from build123d import *

# Parameters (mm, degrees)
BOSS_EXTRUDE1_DEPTH = 10
CHAMFER1_SIZE       = 7.802060087
CHAMFER1_SIZE_2     = 10
BOSS_EXTRUDE2_DEPTH = 20
SKETCH7_R           = 1.5
CUT_EXTRUDE1_DEPTH  = 20
CUT_EXTRUDE3_DEPTH  = 20
FILLET5_R           = 20
FILLET6_R           = 10
SKETCH10_W          = 5.3
SKETCH10_H          = 4.24
CUT_EXTRUDE4_DEPTH  = 273.805653344
SKETCH11_W          = 3.75
SKETCH11_H          = 144.691495626
CUT_EXTRUDE5_DEPTH  = 370.011076387
BOSS_EXTRUDE4_DEPTH = 12.5
SKETCH12_W          = 2
SKETCH12_H          = 1.5
CUT_EXTRUDE6_DEPTH  = 144.691496
CUT_EXTRUDE7_DEPTH  = 273.805653344
SKETCH15_W          = 8
SKETCH15_H          = 10
CUT_EXTRUDE8_DEPTH  = 234.574560204
SKETCH16_R          = 1.45
CUT_EXTRUDE9_DEPTH  = 230.270963046


with BuildPart() as part:
    # Sketch2 → Boss-Extrude1 (new, symmetric)
    with BuildSketch(Plane(origin=(0, 0, 0), x_dir=(0, 0, -1), z_dir=(1, 0, 0))):
        Polygon((36.072931518, 122.5), (-51.279924706, -117.5), (-51.279924706, -192), (-46.279924706, -192), (-46.279924706, -151.5), (-39.679924706, -151.5), (-39.679924706, -192), (-35.679924706, -192), (-35.679924706, -117.5), (-42.766502526, -117.5), (42.766502526, 117.5), (192.766502526, 117.5), (192.766502526, 122.5), align=None)
    extrude(amount=BOSS_EXTRUDE1_DEPTH, both=True)

    # Chamfer1
    # the kernel refuses this chamfer: 10, 7.802060087 mm, written as the material it adds along each edge
    with BuildSketch(Plane(origin=(-10, -117.5, 42.766502526), x_dir=(0, 0.9542611885293297, -0.298974219735734), z_dir=(1, 0, 0))) as chamfer1_piece_1_section:
        Polygon((CHAMFER1_SIZE * 0.998967402661, -CHAMFER1_SIZE * 0.0454326803806), (CHAMFER1_SIZE_2 * 0.298974219736, -CHAMFER1_SIZE_2 * 0.954261188529), (0, 0), align=None)
    chamfer1_piece_1 = extrude(amount=20, mode=Mode.PRIVATE)
    chamfer1_piece_1 = split(chamfer1_piece_1, bisect_by=Plane(origin=(0, -114.855220314, 35.679924706), z_dir=(0, 0, 1)), keep=Keep.TOP, mode=Mode.PRIVATE)
    add(chamfer1_piece_1)

    # Sketch6 → Boss-Extrude2 (add)
    with BuildSketch(Plane(origin=(10, 0, 0), x_dir=(0, 0, -1), z_dir=(1, 0, 0))):
        Polygon((-51.279924706, -180), (-66.279924706, -192), (-51.279924706, -192), align=None)
        Polygon((-35.679924706, -192), (-20.679924706, -192), (-35.679924706, -180), align=None)
    extrude(amount=-BOSS_EXTRUDE2_DEPTH)

    # Sketch7 → Cut-Extrude1 (cut)
    with BuildSketch(Plane(origin=(0, -192, 0), x_dir=(-1, 0, 0), z_dir=(0, -1, 0))):
        with Locations(Location((0, -56.279924706, 0), (0, 0, 90))):
            Circle(SKETCH7_R)
        with Locations(Location((0, -30.179924706, 0), (0, 0, 90))):
            Circle(SKETCH7_R)
    extrude(amount=-CUT_EXTRUDE1_DEPTH, mode=Mode.SUBTRACT)

    # Sketch9 → Cut-Extrude3 (cut)
    with BuildSketch(Plane(origin=(0, -187, 0), x_dir=(-1, 0, 0), z_dir=(0, -1, 0))):
        Polygon((2.75, -57.867637946), (2.75, -54.692211466), (0, -53.104498226), (-2.75, -54.692211466), (-2.75, -57.867637946), (0, -59.455351187), align=None)
        Polygon((2.75, -31.767637946), (2.75, -28.592211466), (0, -27.004498226), (-2.75, -28.592211466), (-2.75, -31.767637946), (0, -33.355351187), align=None)
    extrude(amount=-CUT_EXTRUDE3_DEPTH, mode=Mode.SUBTRACT)

    # Fillet5
    fillet5_edges = [part.edges().sort_by_distance(p)[0] for p in [
        (0, -117.5, 51.279924706),
    ]]
    fillet(fillet5_edges, radius=FILLET5_R)

    # Fillet6
    fillet6_edges = [part.edges().sort_by_distance(p)[0] for p in [
        (0, 122.5, -36.072931518),
    ]]
    fillet(fillet6_edges, radius=FILLET6_R)

    # Sketch10 → Cut-Extrude4 (cut, through all)
    with BuildSketch(Plane(origin=(10, 0, 0), x_dir=(0, 0, -1), z_dir=(1, 0, 0))):
        with Locations((-63.629924706, -189.88)):
            Rectangle(SKETCH10_W, SKETCH10_H)
        with Locations((-23.329924706, -189.88)):
            Rectangle(SKETCH10_W, SKETCH10_H)
    extrude(amount=-CUT_EXTRUDE4_DEPTH, mode=Mode.SUBTRACT)

    # Sketch11 → Cut-Extrude5 (cut, through all)
    with BuildSketch(Plane(origin=(0, 122.5, 0), x_dir=(1, 0, 0), z_dir=(0, 1, 0))):
        with Locations((-8.125, 120.420754713)):
            Rectangle(SKETCH11_W, SKETCH11_H)
        with Locations((8.125, 120.420754713)):
            Rectangle(SKETCH11_W, SKETCH11_H)
    extrude(amount=-CUT_EXTRUDE5_DEPTH, mode=Mode.SUBTRACT)

    # Sketch13 → Boss-Extrude4 (add)
    with BuildSketch(Plane(origin=(6.25, 0, 0), x_dir=(0, 0, -1), z_dir=(1, 0, 0))):
        Polygon((52.766502526, 117.5), (37.766502526, 103.762612903), (42.766502526, 117.5), align=None)
    extrude(amount=-BOSS_EXTRUDE4_DEPTH)

    # Sketch12 → Cut-Extrude6 (cut)
    with BuildSketch(Plane(origin=(0, 0, -192.766502526), x_dir=(-1, 0, 0), z_dir=(0, 0, -1))):
        with Locations((-5.25, 120)):
            Rectangle(SKETCH12_W, SKETCH12_H)
        with Locations((5.25, 120)):
            Rectangle(SKETCH12_W, SKETCH12_H)
    extrude(amount=-CUT_EXTRUDE6_DEPTH, mode=Mode.SUBTRACT)

    # Sketch14 → Cut-Extrude7 (cut, through all)
    with BuildSketch(Plane(origin=(10, 0, 0), x_dir=(0, 0, -1), z_dir=(1, 0, 0))):
        Polygon((-7.517540966, 2.736161147), (0, 0), (0, -210.65241273), (-80.454600392, -210.65241273), (-80.454600392, -132.997640023), align=None)
    extrude(amount=-CUT_EXTRUDE7_DEPTH, mode=Mode.SUBTRACT)

    # Sketch15 → Cut-Extrude8 (cut, through all)
    with BuildSketch(Plane(origin=(0, 2.736161147, 7.517540966), x_dir=(1, 0, 0), z_dir=(0, 0.3420201433256657, 0.9396926207859096))):
        with Locations((0, 5)):
            Rectangle(SKETCH15_W, SKETCH15_H)
    extrude(amount=-CUT_EXTRUDE8_DEPTH, mode=Mode.SUBTRACT)

    # Sketch16 → Cut-Extrude9 (cut, through all)
    with BuildSketch(Plane(origin=(10, 0, 0), x_dir=(0, 0, -1), z_dir=(1, 0, 0))):
        with Locations((-2.048669767, 6.066543677)):
            Circle(SKETCH16_R)
    extrude(amount=-CUT_EXTRUDE9_DEPTH, mode=Mode.SUBTRACT)


solid = part.part
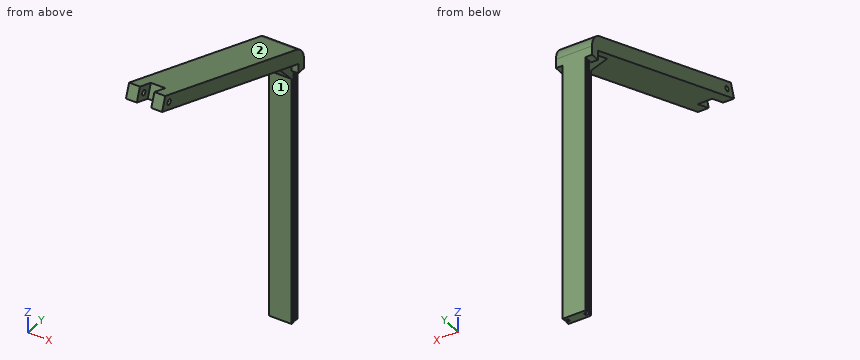
Design review of the part built by this model. Coordinates are the model's own, in mm. Face numbers are marked on the shaded views. A direction names the side the tool comes from. Coordinates: 2 decimals unless noted, no trailing zeros. Loops run counter-clockwise (first coordinate to the right, second up) from the corner with the lowest first, then second, coordinate; pieces in that order, holes last.
Item 1: Add section D-D (y = 92). Write out the cut boundary in (x, z).
Completed:
outline: (-10, -33.49) - (10, -33.49) - (10, -24.97) - (-10, -24.97) - close
Item 2: Add section C-C (y = 109). Write out the cut boundary in (x, z).
Completed:
outline: (-10, -39.67) - (-6.25, -39.67) - (-6.25, -43.49) - (6.25, -43.49) - (6.25, -39.67) - (10, -39.67) - (10, -31.16) - (-10, -31.16) - close
Item 3: Add section A-A (x = -0.5). Write out the cut boundary in (y, z) (1 decimal).
Completed:
outline: (9.4, -3.4) - (103.8, -37.8) - (117.5, -52.8) - (117.5, -192.8) - (122.5, -192.8) - (122.5, -43.1) arc R10 ccw to (115.9, -33.7) - (12.1, 4.1) - close
Item 4: Add section B-B (z = -124). Write out the cut boundary in (x, y).
Completed:
outline: (-6.25, 117.5) - (6.25, 117.5) - (6.25, 119.25) - (4.25, 119.25) - (4.25, 120.75) - (6.25, 120.75) - (6.25, 122.5) - (-6.25, 122.5) - (-6.25, 120.75) - (-4.25, 120.75) - (-4.25, 119.25) - (-6.25, 119.25) - close
Item 5: Clearance check with flat-ended pins moving along their axes: pin 1 (2.5 mm diameter, centred on y = 6.07, z = 2.05, fed in from +X); pin 2 (4 mm diameter, centred on x = -0.5, z = -145, fed in from -Y); pin 3 (8 mm diameter, centred on x = -3, y = 94.5, fed in from +Z); pin 4 (1.2 mm diameter, centred on y = 120.5, z = -106, fed in from +X). State where each tip first meets the part, or that it passes through.
Completed:
pin 1: passes through
pin 2: stops at y = 117.5
pin 3: stops at z = -24.43
pin 4: stops at x = 6.25
Item 6: For the marked faces 1 and 2, list the 3-axis set-ups (+Z, -Z, +X, -X, +Y, -Y) from which the entire face can be reached by the end or side of a thin tool; tool diameter is ignored.
Completed:
face 1: -Z, +X, -X, -Y
face 2: +Z, +X, -X, +Y
Item 7: Wall thickness on L1, parallel to Y at x = 5.5, z = -73; L2, parallel to Y at x = 3.5, z = -131; L3, parallel to Z at x = -1.25, y = 103: over which ranges is each line inside the solid? List them lowest first.
Completed:
L1: y = 117.5 to 119.25, 120.75 to 122.5
L2: y = 117.5 to 122.5
L3: z = -37.49 to -28.98
